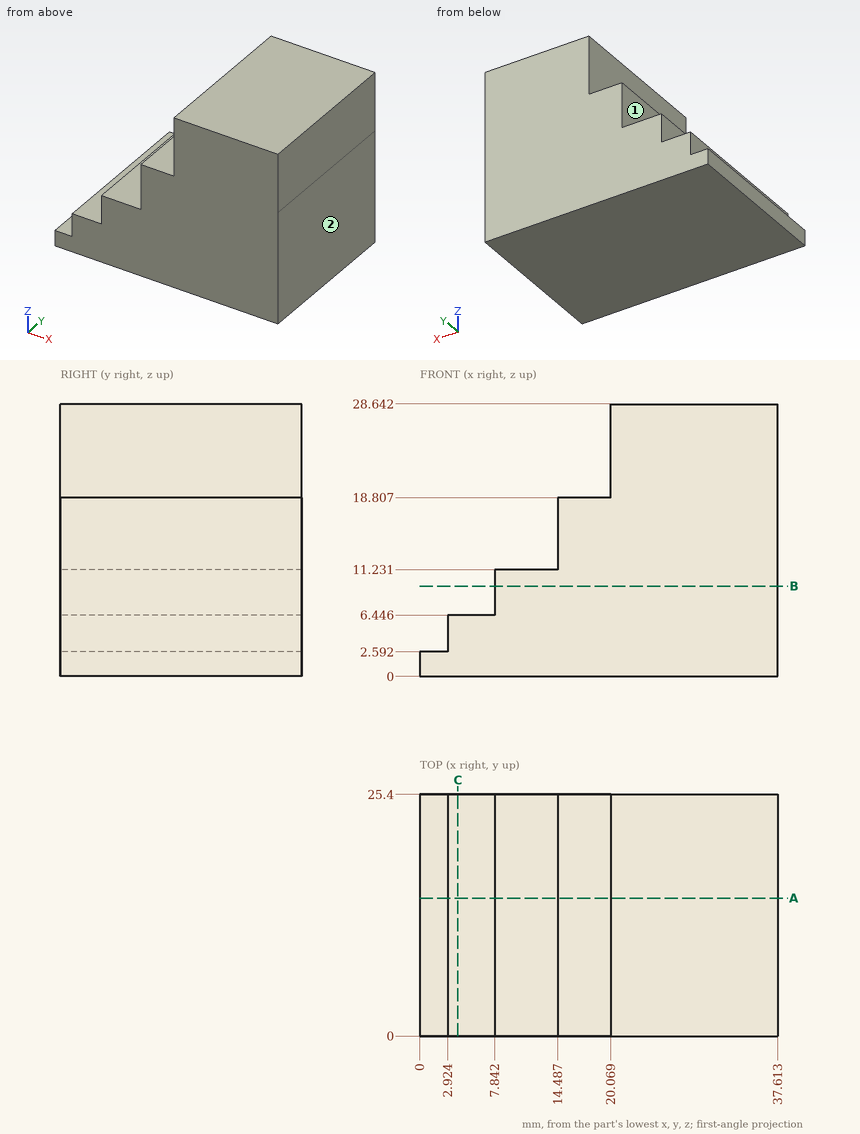
Drawing for the job (mm, zero at the part's lowest x, y, z). A direction names the side the tool comes from. Coordinates: 2 decimals unless noted, no trailing zeros. Loops run counter-clockwise (first coordinate to the right, second up) from the corner with the lowest first, then second, coordinate; pieces in that order, holes last. Notation, with made-up numbers: (-40, 80) - (-7, 80) arc R35 cw to (-7, 113) - close; hole circle Ø10 at (-32, -15.5). An arc over 180 degrees is marked (long way). Return JSON: item names as keys, results as strings.
1. Band-saw the part on B-B (z = 9.5). Give the cut face in (x, y).
Result:
{"outline": "(7.84, 0) - (37.61, 0) - (37.61, 25.4) - (7.84, 25.4) - close"}
2. Band-saw the part on C-C (x = 4). Give the cut face in (y, z).
Result:
{"outline": "(0, 0) - (25.4, 0) - (25.4, 6.45) - (0, 6.45) - close"}
3. Drop flat-ended pins along their axis: pin 1 (3 mm diameter, centred on x = 1, y = 18, fed in from +Z); pin 2 (1.5 mm diameter, centred on x = 19, y = 8, fed in from +Z); pin 3 (2.5 mm diameter, centred on y = 9, z = 14.5, fed in from -X). Give the stop position or say it passes through.
Result:
{"pin 1": "stops at z = 2.59", "pin 2": "stops at z = 18.81", "pin 3": "stops at x = 14.49"}
4. 3-axis set-ups, long thin cutter, end or side, ignore diameter. For the marked faces 1 and 2: which of +Z, -Z, +X, -X, +Y, -Y reach the whole face in a straight line?
Result:
{"face 1": "+Z, -X, +Y, -Y", "face 2": "+Z, -Z, +X, +Y, -Y"}
5. Band-saw the part on A-A (y = 14.5). Give the cut face in (x, z).
Result:
{"outline": "(0, 0) - (37.61, 0) - (37.61, 28.64) - (20.07, 28.64) - (20.07, 18.81) - (14.49, 18.81) - (14.49, 11.23) - (7.84, 11.23) - (7.84, 6.45) - (2.92, 6.45) - (2.92, 2.59) - (0, 2.59) - close"}
6. Probe L1, parallel to X at y = 24, z = 16.25; L2, parallel to Z at x = 16, y = 16.5; L3, parallel to Z at x = 10, y = 13.5. List the from-to ranges inside material, lowest first. Write a range as from..to.
Result:
{"L1": "x = 14.49..37.61", "L2": "z = 0..18.81", "L3": "z = 0..11.23"}
